Input: dimensioned drawing with shaded views. Units: mm. Origin: part minimum x, y, z. Round coordinates to 2 decimals unless told otherwise and drop trailing zeros. Write each loop counter-clockwise with the first axis right and the second up, starting at its lowest first coordinate (ties: lowest second). Pieces come first, ordered by that corner, then holes. Notation, with made-up numbers: (37, 45.5) -> (51, 45.5) arc R12 cw to (51, 60.5) -> close; hole circle Ø7 at (55, -20.5). An arc over 180 degrees is marked (long way). One line per item, written item: value. Start each with the question number.
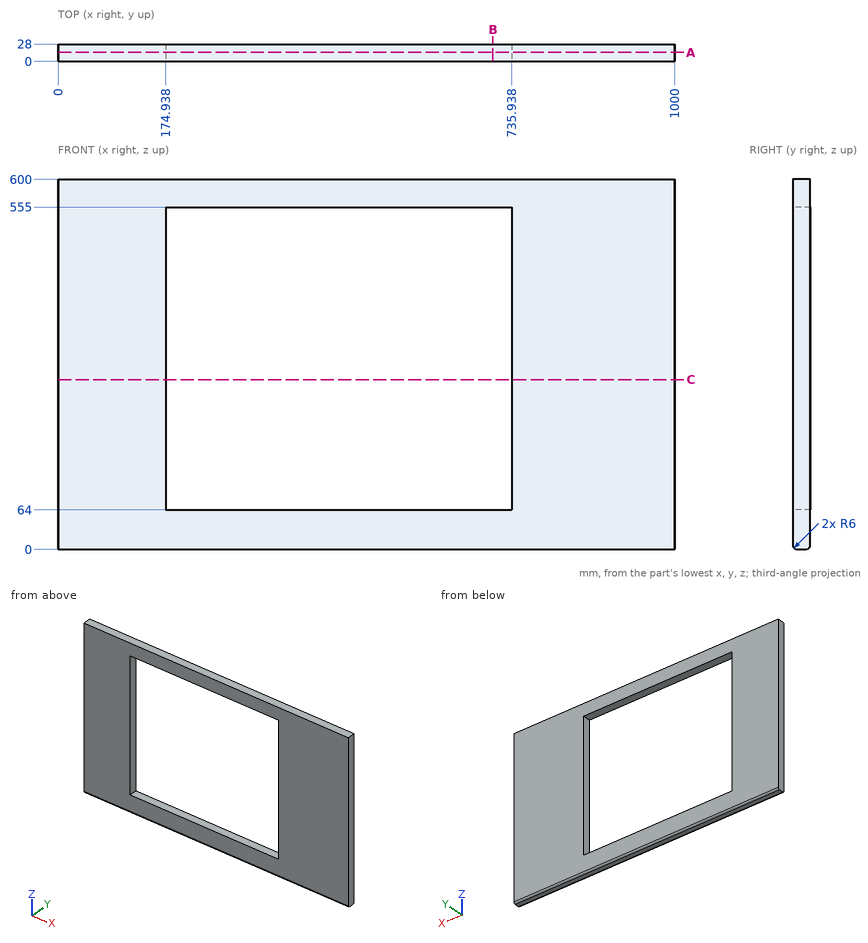
(1) Line query: probe 1 along X at (y, z) = (26.5, 301); probe 2 along Z at (x, y) = (369.5, 10.75); probe 3 along Z at (x, y) = (427.5, 4.75). Output: solid intervals per line, ascending.
(2) Section query B-B (x = 705). Output: boundary loops of the cut face in (y, z).
(3) Pin query (flat end, axial travel): pin 1 (2 mm diameter, centred on x = 104, y = 24.5, fed in from -Z). Return the tip coordinate at first contact, or that it passes through.
(4) Section query C-C (z = 275). Output: boundary loops of the cut face in (x, y).
(5) Section query A-A (y = 14.25). Output: boundary loops of the cut face in (x, z).
Results list:
1. probe 1: x = 0 to 174.94, 735.94 to 1000
1. probe 2: z = 0 to 64, 555 to 600
1. probe 3: z = 0.13 to 64, 555 to 600
2. outline: (0, 6) arc R6 ccw to (6, 0) -> (22, 0) arc R6 ccw to (28, 6) -> (28, 64) -> (0, 64) -> close; (0, 555) -> (28, 555) -> (28, 600) -> (0, 600) -> close
3. pin 1: stops at z = 0.19
4. outline: (0, 0) -> (174.94, 0) -> (174.94, 28) -> (0, 28) -> close; (735.94, 0) -> (1000, 0) -> (1000, 28) -> (735.94, 28) -> close
5. outline: (0, 0) -> (1000, 0) -> (1000, 600) -> (0, 600) -> close; hole (174.94, 64) -> (735.94, 64) -> (735.94, 555) -> (174.94, 555) -> close
